Could you check a few things on this model? Use its own coordinates, in mm. Face numbers are marked on the shaded views. Coordinates: 2 decimals unless noted, no trailing zeros. Order: outer loops, then holes, each group sorted by start corner. A loop starts at its lowest first (then second) coordinate and runs counter-clockwise, first axis right, second up. Notation, with made-up numbers: M -37.75,85 L -0.75,85 A22 cw -0.75,105 Z; hole C 58.5,45 d11. An arc over 180 degrees is marked long. Write item = value, one per line. Start each with the question number.
from build123d import *

# Parameters (mm, degrees)
BOSS_EXTRUDE1_DEPTH = 2
SKETCH2_W           = 2
SKETCH2_H           = 60
BOSS_EXTRUDE2_DEPTH = 50
SKETCH6_R           = 2.5
CUT_EXTRUDE3_DEPTH  = 20
SKETCH8_R           = 2.5
CUT_EXTRUDE5_DEPTH  = 10
SKETCH9_W           = 230
SKETCH9_H           = 50
BOSS_EXTRUDE3_DEPTH = 2
SKETCH10_R          = 2.5
CUT_EXTRUDE6_DEPTH  = 16
SKETCH12_R          = 5
CUT_EXTRUDE7_DEPTH  = 242
SKETCH15_R          = 2.5
CUT_EXTRUDE8_DEPTH  = 242


with BuildPart() as part:
    # Sketch1 → Boss-Extrude1 (new body)
    with BuildSketch(Plane(origin=(0, 0, 0), x_dir=(1, 0, 0), z_dir=(0, 1, 0))):
        Polygon((115, 50), (115, 80), (-115, 80), (-115, 50), (-115, -50), (-115, -75), (115, -75), (115, -50), align=None)
    extrude(amount=BOSS_EXTRUDE1_DEPTH)

    # Sketch2 → Boss-Extrude2 (add)
    with BuildSketch(Plane(origin=(0, 2, 0), x_dir=(1, 0, 0), z_dir=(0, 1, 0))):
        with Locations((-114, 0)):
            Rectangle(SKETCH2_W, SKETCH2_H)
        with Locations((114, 0)):
            Rectangle(SKETCH2_W, SKETCH2_H)
    extrude(amount=BOSS_EXTRUDE2_DEPTH)

    # Sketch6 → Cut-Extrude3 (cut)
    with BuildSketch(Plane(origin=(0, 2, 0), x_dir=(1, 0, 0), z_dir=(0, 1, 0))):
        with Locations(Location((-20, 47.5, 0), (0, 0, 270))):
            Circle(SKETCH6_R)
        with Locations(Location((20, 47.5, 0), (0, 0, 270))):
            Circle(SKETCH6_R)
    extrude(amount=-CUT_EXTRUDE3_DEPTH, mode=Mode.SUBTRACT)

    # Sketch8 → Cut-Extrude5 (cut)
    with BuildSketch(Plane(origin=(0, 2, 0), x_dir=(1, 0, 0), z_dir=(0, 1, 0))):
        with Locations(Location((-20, -32.5, 0), (0, 0, 270))):
            Circle(SKETCH8_R)
        with Locations(Location((20, -32.5, 0), (0, 0, 270))):
            Circle(SKETCH8_R)
    extrude(amount=-CUT_EXTRUDE5_DEPTH, mode=Mode.SUBTRACT)

    # Sketch9 → Boss-Extrude3 (add)
    with BuildSketch(Plane(origin=(0, 2, 0), x_dir=(1, 0, 0), z_dir=(0, 1, 0))):
        with Locations((0, 105)):
            Rectangle(SKETCH9_W, SKETCH9_H)
    extrude(amount=-BOSS_EXTRUDE3_DEPTH)

    # Sketch10 → Cut-Extrude6 (cut)
    with BuildSketch(Plane(origin=(0, 2, 0), x_dir=(1, 0, 0), z_dir=(0, 1, 0))):
        with Locations(Location((-25, 85, 0), (0, 0, 270))):
            Circle(SKETCH10_R)
        with Locations(Location((-25, 105, 0), (0, 0, 270))):
            Circle(SKETCH10_R)
        with Locations(Location((25, 105, 0), (0, 0, 90))):
            Circle(SKETCH10_R)
        with Locations(Location((25, 85, 0), (0, 0, 90))):
            Circle(SKETCH10_R)
    extrude(amount=-CUT_EXTRUDE6_DEPTH, mode=Mode.SUBTRACT)

    # Sketch12 → Cut-Extrude7 (cut)
    with BuildSketch(Plane.ZY.offset(115)):
        with Locations((0, 35.05138551)):
            Circle(SKETCH12_R)
    extrude(amount=-CUT_EXTRUDE7_DEPTH, mode=Mode.SUBTRACT)

    # Sketch15 → Cut-Extrude8 (cut)
    with BuildSketch(Plane.ZY.offset(115)):
        with Locations((-17.223737456, 35)):
            Circle(SKETCH15_R)
        with Locations((17.063876513, 35)):
            Circle(SKETCH15_R)
    extrude(amount=-CUT_EXTRUDE8_DEPTH, mode=Mode.SUBTRACT)


solid = part.part
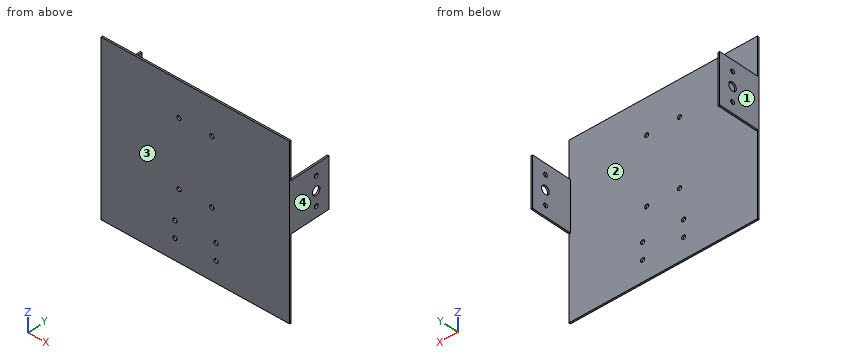
(1) Imagine slicing it at B-B on y = 19.5. List the corners of the cut face in (x, z) for me, plus the area to 3 significant figures.
(2) Imagine slicing it at A-A on x = 25. List the corners of the cut face in (y, z) for me, plus the area to 3 significant figures.
(3) Thinking about a two-plate mould opening in X: for the marked faces 1, 2, 3 and 4, which applies, released by +X, released by -X, zero draft, split by the parting line, or undercut?
(4) Please list where these lines run through material, in increasing order: probe 1 along X at (y, z) = (1.15, -47.5); probe 2 along X at (y, z) = (11.5, -17); probe 3 along X at (y, z) = (1, 32). Write a range as from..to.
(5) Imagine slicing it at C-C on z = 0. List the corners of the cut face in (x, y) for me, plus the area to 3 significant figures.
(6) Will these pins go through, and if not, where does the flat tip stop? P1, Ø6.5, axis at x = -25, z = -85, coming from the +Y side; P2, Ø1, axis at x = -114, y = 30, coming from the +Z side; P3, Ø8, axis at y = 35, z = -17.22, coming from the +X side; P4, Ø1.6, axis at x = 114, y = 20, coming from the -Z side.
(7) Imagine slicing it at D-D on z = -47.5. List the corners of the cut face in (x, y) for me, plus the area to 3 significant figures.
Response:
q1.outline = M -115,-30 L -113,-30 L -113,30 L -115,30 Z; M 113,-30 L 115,-30 L 115,30 L 113,30 Z
q1.area = 240 mm2
q2.outline = M 0,-130 L 2,-130 L 2,-107.5 L 0,-107.5 Z; M 0,-102.5 L 2,-102.5 L 2,-87.5 L 0,-87.5 Z; M 0,-82.5 L 2,-82.5 L 2,75 L 0,75 Z
q2.area = 390 mm2
q3.face_1 = released by -X
q3.face_2 = undercut
q3.face_3 = zero draft
q3.face_4 = released by +X
q4.probe_1 = -115..-22.5, -17.5..17.5, 22.5..115
q4.probe_2 = -115..-113, 113..115
q4.probe_3 = -115..-22.45, -17.55..17.55, 22.45..115
q5.outline = M -115,0 L 115,0 L 115,30.05 L 113,30.05 L 113,2 L -113,2 L -113,30.05 L -115,30.05 Z; M -115,40.05 L -113,40.05 L -113,52 L -115,52 Z; M 113,40.05 L 115,40.05 L 115,52 L 113,52 Z
q5.area = 620 mm2
q6.P1 = 2
q6.P2 = 30
q6.P3 = 115
q6.P4 = -30
q7.outline = M -115,0 L -22.5,0 L -22.5,2 L -115,2 Z; M -17.5,0 L 17.5,0 L 17.5,2 L -17.5,2 Z; M 22.5,0 L 115,0 L 115,2 L 22.5,2 Z
q7.area = 440 mm2
